The listing builds one solid part. Answer for the finished solid, in the listing's coordinates (mm). Face numbers are marked on the shaded views. A direction names the side the tool comes from. Round coordinates to 2 decimals unless told otherwise and drop trailing zeros. Write each loop counter-clockwise with the first axis right and the second up, starting at its lowest first coordinate (ties: lowest second). Pieces come first, ordered by that corner, then holes. Notation, with made-up numbers: M 18,5.25 L 74,5.25 A28 cw 74,32.25 Z; hole C -29,7 d10. An arc over 180 degrees is marked long. One line per item, written item: value. Start each with the question number.
(1) Section D-D (y = -792.5) is taken. Determine the outline of the cut face in (x, z), plus the area to 3 significant figures.
(2) Given P1, Ø12, axis at x = -657, y = 483, coming from the +Z side; P2, Ø3, axis at x = 52, z = -155.5, coming from the +Y side; P3, Ø1, axis at x = -768.5, y = -121, coming from the -Z side, each flat-ended and moving along its own axis, determine where each tip first touches the part or whether it passes through.
(3) Consider probe 1 along Y at (x, z) = (-441.5, 250.5); probe 2 along Z at (x, y) = (-526, -79); probe 3 along X at (y, z) = (223.5, 178.5). Determine where each line is inside the solid, lowest interval first.
(4) Section B-B (x = 968) is taken. Determine the outline of the cut face in (y, z).
(5) For the marked faces 1, 2, 3 and 4, determine the directions among +Z, -Z, +X, -X, +Y, -Y from which every point of the face is accessible in a straight line to the end or side of a thin tool.
(6) For a pull along Y with two mould halves and no side action, classify the marked faces 5, 6 and 7 as released by +Y, released by -Y, zero draft, split by the parting line, or undercut.
(7) Section C-C (y = 110) is taken. Determine the outline of the cut face in (x, z).
(8) Section A-A (z = 239) is taken. Determine the outline of the cut face in (x, y), plus the area to 3 significant figures.
```python
from build123d import *

# Parameters (mm, degrees)
F0_W     = 2290
F0_H     = 1290
F1_DEPTH = 310
F2_T     = -40
F4_DEPTH = 250
F5_R     = 15


with BuildPart() as f1:
    # F0 (on Top) → F1 (new body)
    with BuildSketch(Plane.XY):
        Rectangle(F0_W, F0_H)
    extrude(amount=F1_DEPTH)

    # F2
    f2_openings = [f1.faces().sort_by_distance(p)[0] for p in [
        (0, 0, 310),
        (1145, 0, 155),
    ]]
    offset(amount=F2_T, openings=f2_openings)

    # F3 (on face) → F4 (join)
    with BuildSketch(Plane.XZ.offset(645)):
        with BuildLine():
            Line((-212.795964, 0), (212.795964, 0))
            ThreePointArc((212.795964, 0), (0, 110.35), (-212.795964, 0))
        make_face()
        with BuildLine():
            ThreePointArc((-212.795964, 0), (-78.678756, -398.176904), (260.35, -150))
            ThreePointArc((260.35, -150), (248.176904, -71.321244), (212.795964, 0))
            Line((212.795964, 0), (-212.795964, 0))
        make_face()
    extrude(amount=F4_DEPTH)

    # F5
    f5_edges = [f1.edges().sort_by_distance(p)[0] for p in [
        (-260.35, -895, -150),
    ]]
    fillet(f5_edges, radius=F5_R)


solid = f1.part
```
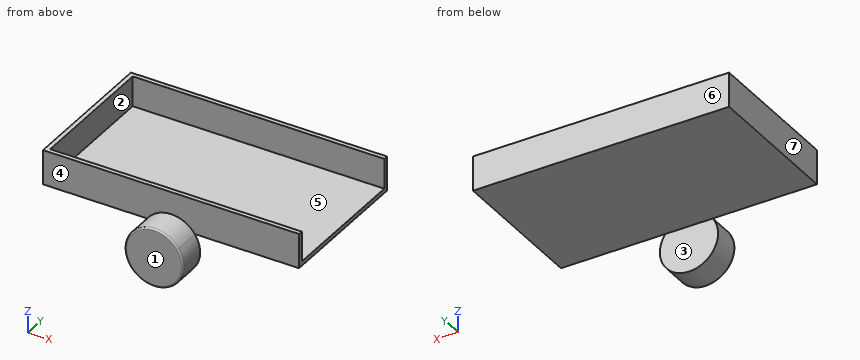
Recorded:
1. outline: M 212.8,0 A260.35 ccw long 260.35,-150 A260.35 ccw Z
1. area: 213,000 mm2
2. P1: stops at z = 40
2. P2: stops at y = -645
2. P3: stops at z = 0
3. probe 1: y = -645 to -605, 605 to 645
3. probe 2: z = 0 to 40
3. probe 3: x = -1145 to -1105
4. outline: M -645,0 L 645,0 L 645,310 L 605,310 L 605,40 L -605,40 L -605,310 L -645,310 Z
5. face 1: +Z, -Z, +X, -X, -Y
5. face 2: +Z, +X
5. face 3: -Z, +X, -X, +Y
5. face 4: +Z, -Y
6. face 5: undercut
6. face 6: released by +Y
6. face 7: zero draft
7. outline: M -1145,0 L 1145,0 L 1145,40 L -1105,40 L -1105,310 L -1145,310 Z
8. outline: M -1145,-645 L 1145,-645 L 1145,-605 L -1105,-605 L -1105,605 L 1145,605 L 1145,645 L -1145,645 Z
8. area: 232,000 mm2
